The listing builds one solid part. Answer for the finished solid, in the listing's coordinates (mm). Face numbers are marked on the shaded views. Round coordinates to 2 decimals unless told otherwise and drop trailing zeros. Write each loop counter-clockwise with the first axis right and the second up, starting at its lowest first coordinate (ties: lowest second). Pieces come first, ordered by that corner, then holes. Notation, with made-up numbers: (2.5, 37) - (54.5, 37) arc R38 ccw to (54.5, 75) - close; hole circle Ø7 at (15.5, 50.5). An arc over 180 degrees is marked (long way). Return JSON: item names as keys, results as strings. Group by question number.
(1) This flat-tipped pin is pushed along its axis until it touches: pin 1 (4 mm diameter, centred on x = -12.5, y = 3, fed in from -Z). Where does it stop, or does it pass through?
(2) Section A-A, the plane y = 0 is taken. Write down the section's boundary in (x, z) (3 decimals), then the cut area to 3 significant figures.
(3) Find the intervals of material crossed by line 1 along Y through (x, z) = (0, 1.3); line 2 along X through (y, z) = (1, 0.65); line 3 along Y through (x, z) = (2, 1), in increasing order. Write a range as [from, to].
(4) Section B-B, the plane x = 0 is taken. Write down the section's boundary in (y, z) (3 decimals).
(5) Section D-D, the plane z = 1.6 is taken. Give the number of separate pieces and of enclosed holes in the cut face, then the cut area to 3 significant figures.
(6) Section C-C, the plane y = 6.5 is taken. Write down the section's boundary in (x, z) (3 decimals).
(7) Determine the mould class of the marked faces 1, 2 and 3 for opening direction Y: +Y half, -Y half, draft (parallel to the pull), parting line (faces both ways), or undercut.
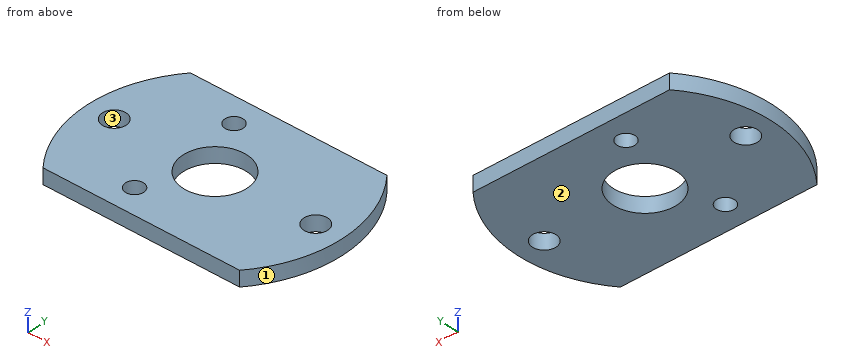
```python
from build123d import *

# Parameters (mm, degrees)
SKETCH1_R             = 15.875
SKETCH1_R_2           = 3.96875
BOSS_EXTRUDE1_DEPTH   = 1.905
MOTORCLEARANCEHOLES_D = 2.9464
ENCODERSETSCREWS_D    = 2.2606
LINACTCUTAWAY_DEPTH   = 23.531317649


with BuildPart() as part:
    # Sketch1 → Boss-Extrude1 (new body)
    with BuildSketch(Plane.XY):
        with Locations(Location((0, 0, 0), (0, 0, 180))):
            Circle(SKETCH1_R)
        with Locations(Location((0, 0, 0), (0, 0, 180))):
            Circle(SKETCH1_R_2, mode=Mode.SUBTRACT)
    extrude(amount=BOSS_EXTRUDE1_DEPTH)

    # MotorClearanceHoles (through all)
    with Locations(Plane.XY.offset(1.905)):
        with Locations((-12.5, 0), (12.5, 0)):
            Hole(MOTORCLEARANCEHOLES_D / 2)

    # EncoderSetScrews (through all)
    with Locations(Plane.XY.offset(1.905)):
        with Locations((-3.81, 6.858), (-3.81, -6.858)):
            Hole(ENCODERSETSCREWS_D / 2)

    # Sketch8 → LinActCutaway (cut, through all)
    with BuildSketch(Plane.XY.offset(1.905)):
        with BuildLine():
            Line((-12.197951672, -10.16), (12.197951672, -10.16))
            ThreePointArc((12.197951672, -10.16), (0, -15.875), (-12.197951672, -10.16))
        make_face()
        with BuildLine():
            Line((-12.197951672, 10.16), (12.197951672, 10.16))
            ThreePointArc((12.197951672, 10.16), (0, 15.875), (-12.197951672, 10.16))
        make_face()
    extrude(amount=-LINACTCUTAWAY_DEPTH, mode=Mode.SUBTRACT)


solid = part.part
```
Working result:
{
 "1": {"pin 1": "stops at z = 0"},
 "2": {"outline": "(-15.875, 0) - (-13.973, 0) - (-13.973, 1.905) - (-15.875, 1.905) - close; (-11.027, 0) - (-3.969, 0) - (-3.969, 1.905) - (-11.027, 1.905) - close; (3.969, 0) - (11.027, 0) - (11.027, 1.905) - (3.969, 1.905) - close; (13.973, 0) - (15.875, 0) - (15.875, 1.905) - (13.973, 1.905) - close", "area": "34.1 mm^2"},
 "3": {"line 1": "y = [-10.16, -3.97], [3.97, 10.16]", "line 2": "x = [-15.84, -13.58], [-11.42, -3.84], [3.84, 11.42], [13.58, 15.84]", "line 3": "y = [-10.16, -3.43], [3.43, 10.16]"},
 "4": {"outline": "(-10.16, 0) - (-3.969, 0) - (-3.969, 1.905) - (-10.16, 1.905) - close; (3.969, 0) - (10.16, 0) - (10.16, 1.905) - (3.969, 1.905) - close"},
 "5": {"separate pieces": "1", "enclosed holes": "5", "area": "527 mm^2"},
 "6": {"outline": "(-14.483, 0) - (-4.882, 0) - (-4.882, 1.905) - (-14.483, 1.905) - close; (-2.738, 0) - (14.483, 0) - (14.483, 1.905) - (-2.738, 1.905) - close"},
 "7": {"face 1": "parting line", "face 2": "draft", "face 3": "undercut"}
}
